```python
from build123d import *

# Parameters (mm, degrees)
F0_W     = 76.2
F0_H     = 127
F1_DEPTH = 58.674
F2_W     = 63.5
F2_H     = 25.4
F2_H_2   = 82.300099
F3_DEPTH = 58.166
F4_R     = 5.08


with BuildPart() as f1:
    # F0 (on Front) → F1 (new body)
    with BuildSketch(Plane.XZ):
        Rectangle(F0_W, F0_H)
    extrude(amount=F1_DEPTH)

    # F2 (on face) → F3 (cut)
    with BuildSketch(Plane.XZ.offset(58.674)):
        with Locations((0.089581, 43.692099)):
            Rectangle(F2_W, F2_H)
        with Locations((0.089581, -15.237951)):
            Rectangle(F2_W, F2_H_2)
    extrude(amount=-F3_DEPTH, mode=Mode.SUBTRACT)

    # F4
    f4_edges = [f1.edges().sort_by_distance(p)[0] for p in [
        (38.1, -29.337, -63.5),
        (-38.1, -29.337, -63.5),
        (0, 0, -63.5),
    ]]
    fillet(f4_edges, radius=F4_R)


solid = f1.part
```
Build history of the part. All positions in model axes, mm. A direction names the side the tool comes from. Round coordinates to 2 decimals unless told otherwise and drop trailing zeros. Loops run counter-clockwise (first coordinate to the right, second up) from the corner with the lowest first, then second, coordinate; pieces in that order, holes last.
Item 1: Pin check, flat tip, straight feed: P1, Ø1.5, axis at x = -22.5, z = 44, coming from the -Y side. Stop position of the tip, or through.
Item 2: Saw through at C-C (z = -48). List the corners of the cut face in (x, y).
Item 3: Saw through at B-B (x = 15.5). List the corners of the cut face in (y, z).
Item 4: Drill centre lines: line 1 along Z through (x, y) = (-19.5, -20.5); line 2 along X through (y, z) = (-8.5, 47); line 3 along Z through (x, y) = (-8.5, -3). Where is each one in solid material? Low to high.
Item 5: Two-plate mould, pull along Z, no slides. Class faces 3 (the face through (-1, -29, 63.5)), 4 (the face through (36.572, -29.748, -62.051)), 5 (the face through (0, -0.508, 44)), 6 (the face through (-1, -58.674, 29)): released by +Z, released by -Z, zero draft, split by the parting line, or undercut.
Item 6: Saw through at A-A (y = -20). List the corners of the cut face in (x, z).
Item 7: Which spindle directions (+Z, -Z, +X, -X, +Y, -Y) get a long thin tool onto all of the face, cutting with end or side? Do faces 1 (the face through (-1, 0, 3)), 2 (the face through (0, -30, 56.392)). Say none if no direction does.
Worked answers:
1. P1: stops at y = -0.51
2. outline: (-38.1, -58.67) - (-31.66, -58.67) - (-31.66, -0.51) - (31.84, -0.51) - (31.84, -58.67) - (38.1, -58.67) - (38.1, 0) - (-38.1, 0) - close
3. outline: (-58.67, -63.5) - (-5.08, -63.5) arc R5.08 ccw to (0, -58.42) - (0, 63.5) - (-58.67, 63.5) - (-58.67, 56.39) - (-0.51, 56.39) - (-0.51, 30.99) - (-58.67, 30.99) - (-58.67, 25.91) - (-0.51, 25.91) - (-0.51, -56.39) - (-58.67, -56.39) - close
4. line 1: z = -63.5 to -56.39, 25.91 to 30.99, 56.39 to 63.5
4. line 2: x = -38.1 to -31.66, 31.84 to 38.1
4. line 3: z = -63.05 to -56.39, 25.91 to 30.99, 56.39 to 63.5
5. face 3: released by +Z
5. face 4: released by -Z
5. face 5: undercut
5. face 6: zero draft
6. outline: (-38.1, -58.42) arc R5.08 ccw to (-33.02, -63.5) - (33.02, -63.5) arc R5.08 ccw to (38.1, -58.42) - (38.1, 63.5) - (-38.1, 63.5) - close; hole (-31.66, -56.39) - (31.84, -56.39) - (31.84, 25.91) - (-31.66, 25.91) - close; hole (-31.66, 30.99) - (31.84, 30.99) - (31.84, 56.39) - (-31.66, 56.39) - close
7. face 1: +Z, -Z, +X, -X, +Y
7. face 2: -Y
